Source: CAD feature listing. Evaluate the final solid. Frame: model axes, mm. A direction names the side the tool comes from. Round coordinates to 2 decimals unless told otherwise and drop trailing zeros. Loops run counter-clockwise (first coordinate to the right, second up) from the corner with the lowest first, then second, coordinate; pieces in that order, holes last. Notation, with made-up numbers: (-9.5, 58.5) - (12.5, 58.5) arc R23 ccw to (12.5, 69.5) - close; hole circle Ø4 at (85.25, 81). An arc over 180 degrees is marked (long way). One line per question, with ' | ' between items. Start each with the question number.
1. Cut plane A-A (z = 0). Return loops of the section in (x, y).
2. Ray query, line 1 (Z direction, x = 0, y = 27); line 2 (Y direction, x = 8.5, z = -5); line 3 (Y direction, x = 2, z = -1.5). Return the intervals inside material, ascending.
3. Cut plane B-B (y = 27). Return loops of the section in (x, z).
4. Pin query (flat end, axial travel): pin 1 (2 mm diameter, centred on y = -4, z = -10.5, fed in from +X); pin 2 (4 mm diameter, centred on x = -12.5, y = -3.5, fed in from +Z); pin 3 (1.5 mm diameter, centred on y = -3, z = 9.5, fed in from -X). Return the tip coordinate at first contact, or that it passes through.
5. Cut plane D-D (y = 20.5). Return loops of the section in (x, z).
6. Mould query, pull axis Z, two halves, no side actions, for faces 1 (the cylindrical face through (-16.024, -1.401, -5.046)), 2 (the flat face through (12, 28.65, -7)), 3 (the cylindrical face through (-1.08, 28.16, 4.88)). Classes: pulls with the +Z half, pulls with the -Z half, needs draft (parallel to the pull), parting line crosses it, or undercut.
7. Access query for faces 4 (the flat face through (0, -30.4, 0)), 5 (the flat face through (-14, -30.65, -6)), 6 (the cylindrical face through (-0.867, 29.664, 3.905)). Directions: +Z, -Z, +X, -X, +Y, -Y. A direction counts if a zero-diameter tool reaches every point of the face in a straight line with its end or side. Return the directions, or none.
8. Cut plane C-C (x = 0). Return loops of the section in (y, z).
Autodesk Inventor part; units mm, degrees
ref_plane "YZ Plane" through (0, 0, 0) normal (1, 0, 0) x (0, 1, 0)
ref_plane "XZ Plane" through (0, 0, 0) normal (0, 1, 0) x (-1, 0, 0)
ref_plane "XY Plane" through (0, 0, 0) normal (0, 0, 1) x (1, 0, 0)
sketch "Sketch1" plane through (0, 0, 0) normal (0, 0, 1) x (1, 0, 0)
  line L0 (-16.8, -30.65) -> (0, -30.65)
  line L1 (0, -30.65) -> (0, 30.65)
  line L2 (0, 30.65) -> (-16.8, 30.65)
  line L3 (-16.8, 30.65) -> (-16.8, -30.65)
  point P0 (0, 0)
  point P1 (0, 0)
  dimension "d0" = 16.8
  dimension "d1" = 61.3
revolve "Revolution1" add sketch "Sketch1" angle 360 about axis through (0, -30.65, 0) along (0, 1, 0)
sketch "Sketch2" plane through (0, 30.65, 0) normal (0, 1, 0) x (1, 0, 0)
  circle A0 centre (0, 0) radius 16.8
  circle A1 centre (0, 0) radius 12.5
  circle A2 centre (0, 0) radius 5
  dimension "d3" = 10
  dimension "d4" = 7.5
extrude "Extrusion1" cut sketch "Sketch2" against normal blind 5 contours A1
sketch "Sketch3" plane through (0, 30.65, 0) normal (0, 1, 0) x (1, 0, 0)
  circle A0 centre (0, 0) radius 16.8
  circle A1 centre (0, 0) radius 12.5
extrude "Extrusion2" cut sketch "Sketch3" against normal blind 2
fillet "Fillet1" radius 1 3 edges at (16.8, -30.65, 0) (16.8, 28.65, 0) (-12.5, 28.65, 0)
sketch "Sketch4" plane through (0, 30.65, 0) normal (0, 1, 0) x (1, 0, 0)
  circle A0 centre (0, 0) radius 5
  circle A1 centre (0, 0) radius 4
  dimension "d10" = 1
extrude "Extrusion3" cut sketch "Sketch4" against normal blind 2
chamfer "Chamfer1" distance 2 angle 45 1 edges at (-5, 25.65, 0)
sketch "Sketch5" plane through (0, -30.65, 0) normal (0, -1, 0) x (1, 0, 0)
  circle A0 centre (0, 0) radius 15.8
  circle A1 centre (0, 0) radius 15
  dimension "d16" = 30
extrude "Extrusion4" cut sketch "Sketch5" against normal blind 0.25 contours A1
properties part number "D Cell"
Answers follow:
1) outline: (-16.8, -29.65) arc R1 ccw to (-15.8, -30.65) - (-15, -30.65) - (-15, -30.4) - (15, -30.4) - (15, -30.65) - (15.8, -30.65) arc R1 ccw to (16.8, -29.65) - (16.8, 27.65) arc R1 ccw to (15.8, 28.65) - (13.5, 28.65) arc R1 ccw to (12.5, 27.65) - (12.5, 25.65) - (7, 25.65) - (5, 27.65) - (5, 28.65) - (4, 28.65) - (4, 30.65) - (-4, 30.65) - (-4, 28.65) - (-5, 28.65) - (-5, 27.65) - (-7, 25.65) - (-12.5, 25.65) - (-12.5, 27.65) arc R1 ccw to (-13.5, 28.65) - (-15.8, 28.65) arc R1 ccw to (-16.8, 27.65) - close
2) line 1: z = -16.8 to -12.5, -5.65 to 5.65, 12.5 to 16.8 | line 2: y = -30.4 to 25.65 | line 3: y = -30.4 to 30.65
3) outline: circle Ø33.6 at (0, 0); circle Ø11.3 at (0, 0); hole circle Ø25 at (0, 0)
4) pin 1: stops at x = 13.86 | pin 2: stops at z = 13.11 | pin 3: stops at x = -14.34
5) outline: circle Ø33.6 at (0, 0)
6) face 1: parting line crosses it | face 2: needs draft | face 3: undercut
7) face 4: -Y | face 5: +Z, -Z, +X, -X, -Y | face 6: +Y
8) outline: (-30.65, -15.8) arc R1 ccw to (-29.65, -16.8) - (27.65, -16.8) arc R1 ccw to (28.65, -15.8) - (28.65, -13.5) arc R1 ccw to (27.65, -12.5) - (25.65, -12.5) - (25.65, -7) - (27.65, -5) - (28.65, -5) - (28.65, -4) - (30.65, -4) - (30.65, 4) - (28.65, 4) - (28.65, 5) - (27.65, 5) - (25.65, 7) - (25.65, 12.5) - (27.65, 12.5) arc R1 ccw to (28.65, 13.5) - (28.65, 15.8) arc R1 ccw to (27.65, 16.8) - (-29.65, 16.8) arc R1 ccw to (-30.65, 15.8) - (-30.65, 15) - (-30.4, 15) - (-30.4, -15) - (-30.65, -15) - close
